```python
from build123d import *

# Parameters (mm, degrees)
ESQUISSE1_W             = 16
ESQUISSE1_H             = 12
EXTRUSION1_DEPTH        = 14
CHANFREIN1_SIZE         = 14
ESQUISSE3_R             = 1.5
ENL_V_MAT_EXTRU_2_DEPTH = 24.323807579
TROU_TARAUD_M3X0_51_D   = 2.5


with BuildPart() as part:
    # Esquisse1 → Extrusion1 (new body)
    with BuildSketch(Plane.XY):
        with Locations((8, 6)):
            Rectangle(ESQUISSE1_W, ESQUISSE1_H)
    extrude(amount=EXTRUSION1_DEPTH)

    # Chanfrein1
    # the kernel refuses this chamfer: 14 mm, written as the material it takes off along each edge
    with BuildSketch(Plane(origin=(52.003561832, 12, 14), x_dir=(0, 0.027495876610586365, -0.9996219169112968), z_dir=(-1, 0, 0))) as chanfrein1_piece_1:
        Polygon((CHANFREIN1_SIZE * 0.999621916911, CHANFREIN1_SIZE * 0.0274958766106), (-CHANFREIN1_SIZE * 0.0274958766106, CHANFREIN1_SIZE * 0.999621916911), (0, 0), align=None)
    extrude(amount=88.007123663, mode=Mode.SUBTRACT)

    # Esquisse3 → Enlèv. mat.-Extru.2 (cut, through all)
    with BuildSketch(Plane(origin=(0, 0, 0), x_dir=(-1, 0, 0), z_dir=(0, 0, -1))):
        with Locations((-8, 4)):
            Circle(ESQUISSE3_R)
    extrude(amount=-ENL_V_MAT_EXTRU_2_DEPTH, mode=Mode.SUBTRACT)

    # Trou taraudé M3x0.51 (through all)
    with Locations(Plane(origin=(16, 0, 0), x_dir=(0, 0, -1), z_dir=(1, 0, 0))):
        with Locations((-3.5, 4)):
            Hole(TROU_TARAUD_M3X0_51_D / 2)


solid = part.part
```
For this review, take the finished solid that the model builds, in its own axes (mm). Coordinates: 2 decimals unless noted, no trailing zeros. Loops run counter-clockwise (first coordinate to the right, second up) from the corner with the lowest first, then second, coordinate; pieces in that order, holes last. Notation, with made-up numbers: (73.5, 62.5) -> (82.5, 62.5) arc R18 ccw to (82.5, 93.5) -> close; hole circle Ø11 at (-8.5, -19.5). An arc over 180 degrees is marked (long way). Return JSON: item names as keys, results as strings. Group by question number.
(1) For pin 1 Ø3.5 at (x, y) = (8, 4) entering from -Z; pin 2 Ø3 at (y, z) = (6.5, 9.5) entering from -X, all flat-tipped, find the tip position at first contact; note any pin that passes through.
(2) Consider section B-B, the plane z = 3.5. Give the boundary of the cut face in (x, y).
(3) Mouldability with a two-part tool opening along Z and no side actions: class faces 1 (the flat face through (8, 6, 0)), 2 (the flat face through (8, 0, 6)), 3 (the flat face through (8, 6, 6)), 4 (the cylindrical face through (12.364, 3.521, 4.655)) as pulls with the +Z half, pulls with the -Z half, needs draft (parallel to the pull), parting line crosses it, or undercut.
(4) Consider section A-A, the plane y = 4. Give the boundary of the cut face in (x, z), plus the area to 3 significant figures.
(5) Consider section C-C, the plane x = 8. Give the boundary of the cut face in (y, z).
(6) To check wall thickness, follow L1, parallel to Y at x = 8, z = 5.5; L2, parallel to Z at x = 12.25, y = 4; L3, parallel to Y at x = 4, z = 3.5. State the ranges of each line that lie inside material, in increasing order.
(7) Consider section D-D, the plane z = 9.25. Give the boundary of the cut face in (x, y).
Results below:
{
 "1": {"pin 1": "stops at z = 0", "pin 2": "passes through"},
 "2": {"outline": "(0, 0) -> (16, 0) -> (16, 2.75) -> (8.83, 2.75) arc R1.5 cw to (7.17, 2.75) -> (0, 2.75) -> close; (0, 5.25) -> (7.17, 5.25) arc R1.5 cw to (8.83, 5.25) -> (16, 5.25) -> (16, 8.5) -> (0, 8.5) -> close"},
 "3": {"face 1": "pulls with the -Z half", "face 2": "needs draft", "face 3": "pulls with the +Z half", "face 4": "undercut"},
 "4": {"outline": "(0, 0) -> (6.5, 0) -> (6.5, 2.25) -> (0, 2.25) -> close; (0, 4.75) -> (6.5, 4.75) -> (6.5, 8) -> (0, 8) -> close; (9.5, 0) -> (16, 0) -> (16, 2.25) -> (9.5, 2.25) -> close; (9.5, 4.75) -> (16, 4.75) -> (16, 8) -> (9.5, 8) -> close", "area": "71.5 mm2"},
 "5": {"outline": "(0, 0) -> (2.5, 0) -> (2.5, 9.5) -> (0, 12) -> close; (5.5, 0) -> (12, 0) -> (5.5, 6.5) -> close"},
 "6": {"L1": "y = 0 to 2.5, 5.5 to 6.5", "L2": "z = 0 to 2.25, 4.75 to 8", "L3": "y = 0 to 2.75, 5.25 to 8.5"},
 "7": {"outline": "(0, 0) -> (16, 0) -> (16, 2.75) -> (8.83, 2.75) arc R1.5 cw to (7.17, 2.75) -> (0, 2.75) -> close"}
}
